```python
from build123d import *

# Parameters (mm, degrees)
SZKIC1_W                    = 1200
SZKIC1_H                    = 580
DODANIE_WYCI_GNI_CIE1_DEPTH = 150
SZKIC2_W                    = 1210
SZKIC2_H                    = 590
SZKIC2_W_2                  = 1200
SZKIC2_H_2                  = 580
DODANIE_WYCI_GNI_CIE2_DEPTH = 20
SZKIC3_R                    = 15
DODANIE_WYCI_GNI_CIE3_DEPTH = 10
SZYK_LINIOWY1_COUNT         = 3
SZYK_LINIOWY1_PITCH         = 400
LUSTRO1_COPY_1_SKETCH_R     = 15
LUSTRO1_COPY_1_DEPTH        = 10
LUSTRO1_COPY_2_SKETCH_R     = 15
LUSTRO1_COPY_2_DEPTH        = 10


with BuildPart() as part:
    # Szkic1 → Dodanie-wyciągnięcie1 (new body)
    with BuildSketch(Plane(origin=(0, 0, 0), x_dir=(1, 0, 0), z_dir=(0, 1, 0))):
        with Locations((600, 290)):
            Rectangle(SZKIC1_W, SZKIC1_H)
    extrude(amount=DODANIE_WYCI_GNI_CIE1_DEPTH)

    # Szkic2 → Dodanie-wyciągnięcie2 (add, symmetric)
    with BuildSketch(Plane(origin=(0, 60, 0), x_dir=(1, 0, 0), z_dir=(0, 1, 0))):
        with Locations((600, 290)):
            Rectangle(SZKIC2_W, SZKIC2_H)
        with Locations((600, 290)):
            Rectangle(SZKIC2_W_2, SZKIC2_H_2, mode=Mode.SUBTRACT)
    extrude(amount=DODANIE_WYCI_GNI_CIE2_DEPTH, both=True)

    # Szkic3 → Dodanie-wyciągnięcie3 (add)
    with BuildSketch(Plane.XY.offset(5)):
        with Locations(Location((195, 60, 0), (0, 0, 180))):
            Circle(SZKIC3_R)
    dodanie_wyci_gni_cie3 = extrude(amount=DODANIE_WYCI_GNI_CIE3_DEPTH)

    # Szyk liniowy1: Dodanie-wyciągnięcie3 ×3
    with Locations(*[(i * SZYK_LINIOWY1_PITCH, 0, 0) for i in range(1, SZYK_LINIOWY1_COUNT)]):
        add(dodanie_wyci_gni_cie3)

    # Lustro1: Dodanie-wyciągnięcie3 across plane
    add(dodanie_wyci_gni_cie3.mirror(Plane.XY.offset(-290)))

    # Lustro1 copy 1 sketch → Lustro1 copy 1 (add)
    with BuildSketch(Plane(origin=(400, 0, -585), x_dir=(1, 0, 0), z_dir=(0, 0, -1))):
        with Locations((195, -60)):
            Circle(LUSTRO1_COPY_1_SKETCH_R)
    extrude(amount=LUSTRO1_COPY_1_DEPTH)

    # Lustro1 copy 2 sketch → Lustro1 copy 2 (add)
    with BuildSketch(Plane(origin=(800, 0, -585), x_dir=(1, 0, 0), z_dir=(0, 0, -1))):
        with Locations((195, -60)):
            Circle(LUSTRO1_COPY_2_SKETCH_R)
    extrude(amount=LUSTRO1_COPY_2_DEPTH)


solid = part.part
```
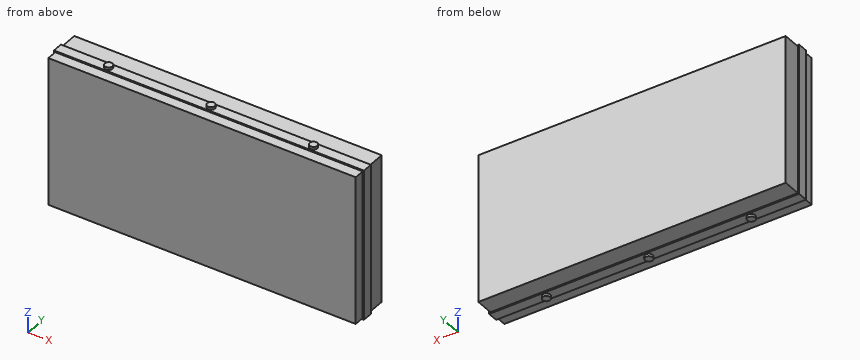
The listing builds one solid part. Answer for the finished solid, in the listing's coordinates (mm). Give positions to 0.01 mm unless a question says otherwise; leave off trailing zeros. Order: outer loops, then holes, each group sorted by start corner. A loop starts at its lowest first (then second) coordinate and runs counter-clockwise, first axis right, second up. Notation, with made-up numbers: (-24.5, -31) - (-19.5, -31) arc R19 ccw to (-19.5, 0) - close; hole circle Ø3 at (-32.5, 81.5). An arc over 180 degrees is marked (long way). Answer in a Markdown table with one row per item. Add a question column.
Q1. The part is cut by section A-A (x = 274). Determine the outline of the cut face in (y, z).
Q2. Given P1, Ø20, axis at x = 856.5, y = 19, coming from the +Z side; P2, Ø5, axis at y = 133, z = -487, coming from the -X side; P3, Ø1.5, axis at x = 201.5, z = -102, coming from the -Y side; P4, Ø2, axis at x = 236, y = 68.5, coming from the -Z side, each flat-ended and moving along its own axis, determine where each tip first touches the part or whether it passes through.
Q3. The part is cut by section C-C (x = 595). Determine the outline of the cut face in (y, z).
Q4. The part is cut by section B-B (y = 60). Determine the outline of the cut face in (x, z).
Q5. Find the intervals of material crossed by line 1 along X through (y, z) = (140.5, -141); line 2 along Z through (x, y) = (731, 32); line 3 along Z through (x, y) = (911.5, 76), in increasing order. Write a range as [from, to].
Determined:
| question | item | result |
|---|---|---|
| 1 | outline | (0, -580) - (40, -580) - (40, -585) - (80, -585) - (80, -580) - (150, -580) - (150, 0) - (80, 0) - (80, 5) - (40, 5) - (40, 0) - (0, 0) - close |
| 2 | P1 | stops at z = 0 |
| 2 | P2 | stops at x = 0 |
| 2 | P3 | stops at y = 0 |
| 2 | P4 | stops at z = -585 |
| 3 | outline | (0, -580) - (40, -580) - (40, -585) - (45, -585) - (45, -595) - (75, -595) - (75, -585) - (80, -585) - (80, -580) - (150, -580) - (150, 0) - (80, 0) - (80, 5) - (75, 5) - (75, 15) - (45, 15) - (45, 5) - (40, 5) - (40, 0) - (0, 0) - close |
| 4 | outline | (-5, -585) - (180, -585) - (180, -595) - (210, -595) - (210, -585) - (580, -585) - (580, -595) - (610, -595) - (610, -585) - (980, -585) - (980, -595) - (1010, -595) - (1010, -585) - (1205, -585) - (1205, 5) - (1010, 5) - (1010, 15) - (980, 15) - (980, 5) - (610, 5) - (610, 15) - (580, 15) - (580, 5) - (210, 5) - (210, 15) - (180, 15) - (180, 5) - (-5, 5) - close |
| 5 | line 1 | x = [0, 1200] |
| 5 | line 2 | z = [-580, 0] |
| 5 | line 3 | z = [-585, 5] |
